```python
from build123d import *

# Parameters (mm, degrees)
F1_DEPTH = 32
F2_R     = 5.5
F4_DEPTH = 13.001
F3_R     = 5.5
F5_DEPTH = 13.001
F7_DEPTH = 88.001
F9_DEPTH = 88.001


with BuildPart() as f1:
    # F0 (on Front) → F1 (new body)
    with BuildSketch(Plane.XZ):
        Polygon((17.5, 0), (56.5, 0), (56.5, 13), (31.5, 13), (31.5, 64), (12.5, 64), (12.5, 30), (-12.5, 30), (-12.5, 64), (-31.5, 64), (-31.5, 13), (-56.5, 13), (-56.5, 0), (-17.5, 0), (-17.5, 17), (17.5, 17), align=None)
    extrude(amount=F1_DEPTH)

    # F2 (on face) → F4 (cut, through all)
    with BuildSketch(Plane.XY.offset(13)):
        with Locations((-44, -16)):
            Circle(F2_R)
    extrude(amount=-F4_DEPTH, mode=Mode.SUBTRACT)

    # F3 (on face) → F5 (cut, through all)
    with BuildSketch(Plane.XY.offset(13)):
        with Locations((44, -16)):
            Circle(F3_R)
    extrude(amount=-F5_DEPTH, mode=Mode.SUBTRACT)

    # F6 (on face) → F7 (cut, through all)
    with BuildSketch(Plane(origin=(-31.5, 0, 0), x_dir=(0, -1, 0), z_dir=(-1, 0, 0))):
        with BuildLine():
            ThreePointArc((22.5, 46), (11.403806, 50.596194), (16, 39.5))
            ThreePointArc((16, 39.5), (20.596194, 41.403806), (22.5, 46))
        make_face()
    extrude(amount=-F7_DEPTH, mode=Mode.SUBTRACT)

    # F8 (on face) → F9 (cut, through all)
    with BuildSketch(Plane(origin=(-31.5, 0, 0), x_dir=(0, -1, 0), z_dir=(-1, 0, 0))):
        with BuildLine():
            ThreePointArc((0, 56), (16, 59.871235), (32, 56))
            Line((32, 56), (32, 64))
            Line((32, 64), (0, 64))
            Line((0, 64), (0, 56))
        make_face()
    extrude(amount=-F9_DEPTH, mode=Mode.SUBTRACT)


solid = f1.part
```
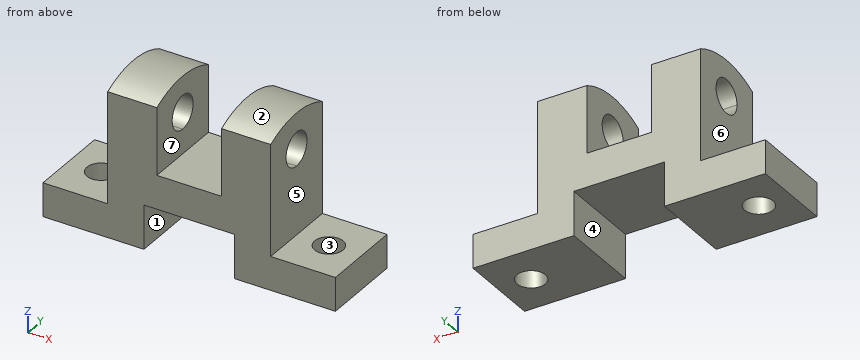
Could you check a few things on this model? Use its own coordinates, in mm. Face numbers are marked on the shaded views. A direction names the side the tool comes from. Round coordinates to 2 decimals unless told otherwise and drop trailing zeros. Loops run counter-clockwise (first coordinate to the right, second up) from the corner with the lowest first, then second, coordinate; pieces in that order, holes last. Notation, with made-up numbers: M 32,63 L 86,63 A10 ccw 86,72 Z; hole C -12,49.5 d10. An arc over 180 degrees is marked long. Put each result on its own line as item: value.
Q1. Thinking about a two-plate mould opening in Y: for the marked faces 1, 2 and 3, which applies, released by +Y, released by -Y, zero draft, split by the parting line, or undercut?
Check result:
face 1: zero draft
face 2: split by the parting line
face 3: undercut
Q2. For pin 1 (17 mm diameter, centred on y = -16, z = 46, fed in from -X); pin 2 (10.5 mm diameter, centred on y = -16, z = 46, fed in from -X); pin 3 (10 mm diameter, centred on x = 31.5, y = -3.5, fed in from +Z); pin 4 (1.5 mm diameter, centred on x = -12, y = -12, fed in from +Z), each with a flat end and sliding along its axis, tell me the tip position at first contact or that it passes through.
Check result:
pin 1: x = -31.5
pin 2: through
pin 3: z = 59.06
pin 4: z = 59.7
Q3. Imagine slicing it at D-D (x = 16). Write out the boundary of the cut face in (y, z), then the cut area to 3 significant figures.
Check result:
outline: M -32,17 L 0,17 L 0,56 A35 ccw -32,56 Z; hole C -16,46 d13
area: 1,200 mm2
Q4. On a 3-axis mill with a long thin cutter (end or side, diameter ignored), from which of +Z, -Z, +X, -X, +Y, -Y can I reach the whole of each face in a straight line? I mean the marked faces 4, 5, 6 and 7. Say none if no direction works.
Check result:
face 4: -Z, +Y, -Y
face 5: +Z, +X, +Y, -Y
face 6: +Z, -X, +Y, -Y
face 7: +Z, +Y, -Y
Q5. Imagine slicing it at A-A (z = 5). Write out the boundary of the cut face in (x, y), then the cut area to 3 significant figures.
Check result:
outline: M -56.5,-32 L -17.5,-32 L -17.5,0 L -56.5,0 Z; M 17.5,-32 L 56.5,-32 L 56.5,0 L 17.5,0 Z; hole C -44,-16 d11; hole C 44,-16 d11
area: 2,310 mm2
Q6. Imagine slicing it at B-B (x = -44). Write out the boundary of the cut face in (y, z), then the cut area to 3 significant figures.
Check result:
outline: M -32,0 L -21.5,0 L -21.5,13 L -32,13 Z; M -10.5,0 L 0,0 L 0,13 L -10.5,13 Z
area: 273 mm2
Q7. Imagine slicing it at C-C (y = -14.5). State how many separate pieces and enclosed holes the cut face has, then the cut area to 3 significant figures.
Check result:
separate pieces: 5
enclosed holes: 0
area: 2,320 mm2
Q8. I need wall thicknesses on probe 1 along X at (y, z) = (-2.5, 47); probe 2 along Y at (x, z) = (19, 46); probe 3 along Y at (x, z) = (44, 3). Which ranges of each line are inside material? Lowest first, please.
Check result:
probe 1: -31.5 to -12.5, 12.5 to 31.5
probe 2: -32 to -22.5, -9.5 to 0
probe 3: -32 to -21.5, -10.5 to 0
